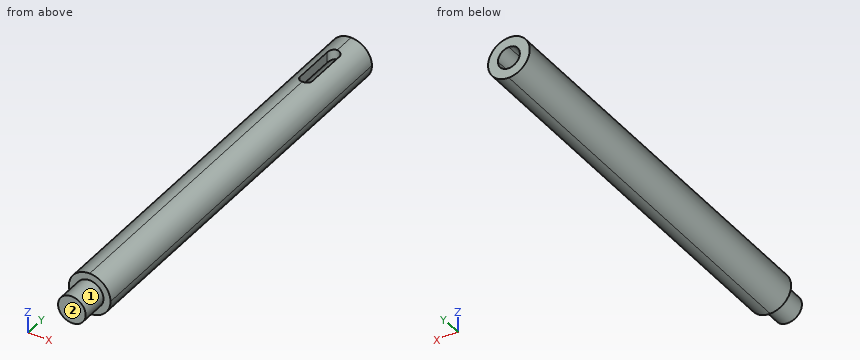
```python
from build123d import *

# Parameters (mm, degrees)
F1_DEPTH = 183
F2_DEPTH = 120
F4_DEPTH = 25
F5_R     = 6.3
F6_DEPTH = 12.5


with BuildPart() as f1:
    # F0 (on Front) → F1 (new body)
    with BuildSketch(Plane.XZ):
        with BuildLine():
            ThreePointArc((0, -9.5), (6.717514, -6.717514), (9.5, 0))
            ThreePointArc((9.5, 0), (6.717514, 6.717514), (0, 9.5))
            Line((0, 9.5), (0, 5))
            ThreePointArc((0, 5), (3.535534, 3.535534), (5, 0))
            ThreePointArc((5, 0), (3.535534, -3.535534), (0, -5))
            Line((0, -5), (0, -9.5))
        make_face()
        with BuildLine():
            ThreePointArc((5, 0), (3.535534, 3.535534), (0, 5))
            Line((0, 5), (0, -5))
            ThreePointArc((0, -5), (3.535534, -3.535534), (5, 0))
        make_face()
        with BuildLine():
            Line((0, -5), (0, 5))
            ThreePointArc((0, 5), (-5, 0), (0, -5))
        make_face()
        with BuildLine():
            Line((0, 5), (0, 9.5))
            ThreePointArc((0, 9.5), (-9.5, 0), (0, -9.5))
            Line((0, -9.5), (0, -5))
            ThreePointArc((0, -5), (-5, 0), (0, 5))
        make_face()
    extrude(amount=F1_DEPTH)

    # F0 (on Front) → F2 (cut)
    with BuildSketch(Plane.XZ):
        with BuildLine():
            ThreePointArc((5, 0), (3.535534, 3.535534), (0, 5))
            Line((0, 5), (0, -5))
            ThreePointArc((0, -5), (3.535534, -3.535534), (5, 0))
        make_face()
        with BuildLine():
            Line((0, -5), (0, 5))
            ThreePointArc((0, 5), (-5, 0), (0, -5))
        make_face()
    extrude(amount=F2_DEPTH, mode=Mode.SUBTRACT)

    # F3 (on Top) → F4 (cut)
    with BuildSketch(Plane.XY):
        with BuildLine():
            Line((2.746924, -31.5), (2.746924, -12.5))
            ThreePointArc((2.746924, -12.5), (-0.003076, -9.75), (-2.753076, -12.5))
            Line((-2.753076, -12.5), (-2.753076, -31.5))
            ThreePointArc((-2.753076, -31.5), (-0.003076, -34.25), (2.746924, -31.5))
        make_face()
    extrude(amount=F4_DEPTH, mode=Mode.SUBTRACT)

    # F5 (on face) → F6 (join)
    with BuildSketch(Plane.XZ.offset(183)):
        Circle(F5_R)
    extrude(amount=F6_DEPTH)


solid = f1.part
```
The model under review builds one solid part; all positions refer to its coordinate system, in mm. Face numbers are marked on the shaded views. A direction names the side the tool comes from. Round coordinates to 2 decimals unless told otherwise and drop trailing zeros. Order: outer loops, then holes, each group sorted by start corner. A loop starts at its lowest first (then second) coordinate and runs counter-clockwise, first axis right, second up. Notation, with made-up numbers: (-15.5, 66.25) -> (15.5, 66.25) arc R15 ccw to (15.5, 72.25) -> close; hole circle Ø6 at (23, 61). An arc over 180 degrees is marked (long way). Use a Markdown table: item, result.
Q1. Tool access review of the marked faces 1 and 2: name each direction out of +Z, -Z, +X, -X, +Y, -Y from which nothing blocks a thin tool from reaching the whole face with its end or side.
Values:
| item | result |
|---|---|
| face 1 | -Y |
| face 2 | +Z, -Z, +X, -X, -Y |
Q2. We need section A-A on y = -71. Write out the cut boundary in (x, z), then the cut area to 3 significant figures.
Values:
| item | result |
|---|---|
| outline | (0, -9.5) arc R9.5 ccw to (9.5, 0) arc R9.5 ccw to (0, 9.5) arc R9.5 ccw to start; hole circle Ø10 at (0, 0) |
| area | 205 mm^2 |
Q3. Clearance check with flat-ended pins moving along their axes: P1, Ø5.5, axis at y = -25, z = 6, coming from the -X side; P2, Ø1.5, axis at x = 3, y = -172.5, coming from the +Z side; P3, Ø5, axis at x = 0, z = -2, coming from the +Y side; P4, Ø4, axis at x = 3, z = -6, coming from the +Y side. State where each tip first meets the part, or that it passes through.
Values:
| item | result |
|---|---|
| P1 | stops at x = -8.93 |
| P2 | stops at z = 9.23 |
| P3 | stops at y = -120 |
| P4 | stops at y = 0 |
Q4. We need section B-B on z = 2.5. Write out the cut boundary in (x, y), then the cut area to 3 significant figures.
Values:
| item | result |
|---|---|
| outline | (-9.17, -183) -> (-5.78, -183) -> (-5.78, -195.5) -> (5.78, -195.5) -> (5.78, -183) -> (9.17, -183) -> (9.17, 0) -> (4.33, 0) -> (4.33, -120) -> (-4.33, -120) -> (-4.33, 0) -> (-9.17, 0) -> close |
| area | 2,460 mm^2 |
Q5. For line 1 (Y direction, x = -0.25, z = 7); line 2 (Y direction, x = -7.25, z = -4.25); line 3 (Z direction, x = 0.25, y = -151.5), list the stretches that pass through material, from the lowest coordinate up.
Values:
| item | result |
|---|---|
| line 1 | y = -183 to -34.24, -9.76 to 0 |
| line 2 | y = -183 to 0 |
| line 3 | z = -9.5 to 9.5 |
